Drawing for the job (mm, zero at the part's lowest x, y, z). Round coordinates to 2 decimals unless told otherwise and drop trailing zeros. Loops run counter-clockwise (first coordinate to the right, second up) from the corner with the lowest first, then second, coordinate; pieces in that order, holes last. Notation, with made-up numbers: M 48,89.25 L 90,89.25 A21 ccw 90,114.25 Z; hole C -8.75,-34 d10. An arc over 180 degrees is marked long. Write each question's results on one line, items separated by ' | '.
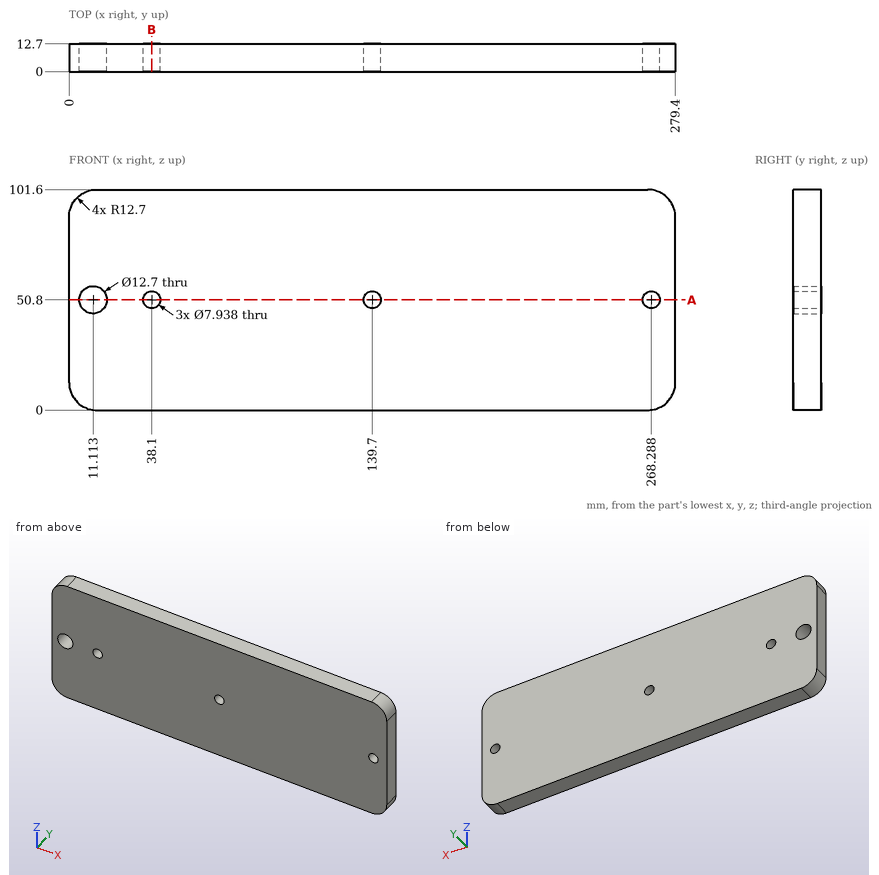
Item 1: Wall check: L1, parallel to Z at x = 139.7, y = 6.25; L2, parallel to X at y = 5.5, z = 90; L3, parallel to X at y = 11.5, z = 95. Give the ranges that are in metal, low to high.
Filled sheet:
L1: 0 to 46.83, 54.77 to 101.6 | L2: 0.05 to 279.35 | L3: 1.56 to 277.84
Item 2: Band-saw the part on A-A on z = 50.8. Give the cut face in (x, y).
Filled sheet:
outline: M 0,0 L 4.76,0 L 4.76,12.7 L 0,12.7 Z; M 17.46,0 L 34.13,0 L 34.13,12.7 L 17.46,12.7 Z; M 42.07,0 L 135.73,0 L 135.73,12.7 L 42.07,12.7 Z; M 143.67,0 L 264.32,0 L 264.32,12.7 L 143.67,12.7 Z; M 272.26,0 L 279.4,0 L 279.4,12.7 L 272.26,12.7 Z
Item 3: Band-saw the part on B-B on x = 38.1. Give the cut face in (y, z), and give its area (3 significant figures).
Filled sheet:
outline: M 0,0 L 12.7,0 L 12.7,46.83 L 0,46.83 Z; M 0,54.77 L 12.7,54.77 L 12.7,101.6 L 0,101.6 Z | area: 1,190 mm^2
